For this review, use the dimensioned drawing (mm, ordinates from the lowest corner) and the shaded views. Coordinates: 2 decimals unless noted, no trailing zeros. Order: outer loops, then holes, each group sorted by start corner. A loop starts at its lowest first (then second) coordinate and runs counter-clockwise, first axis right, second up. Notation, with made-up numbers: M 80.25,69.25 L 103.25,69.25 A21 cw 103.25,86.25 Z; hole C 39.25,-10.75 d7. An arc over 180 degrees is marked long. One line per item, written item: value.
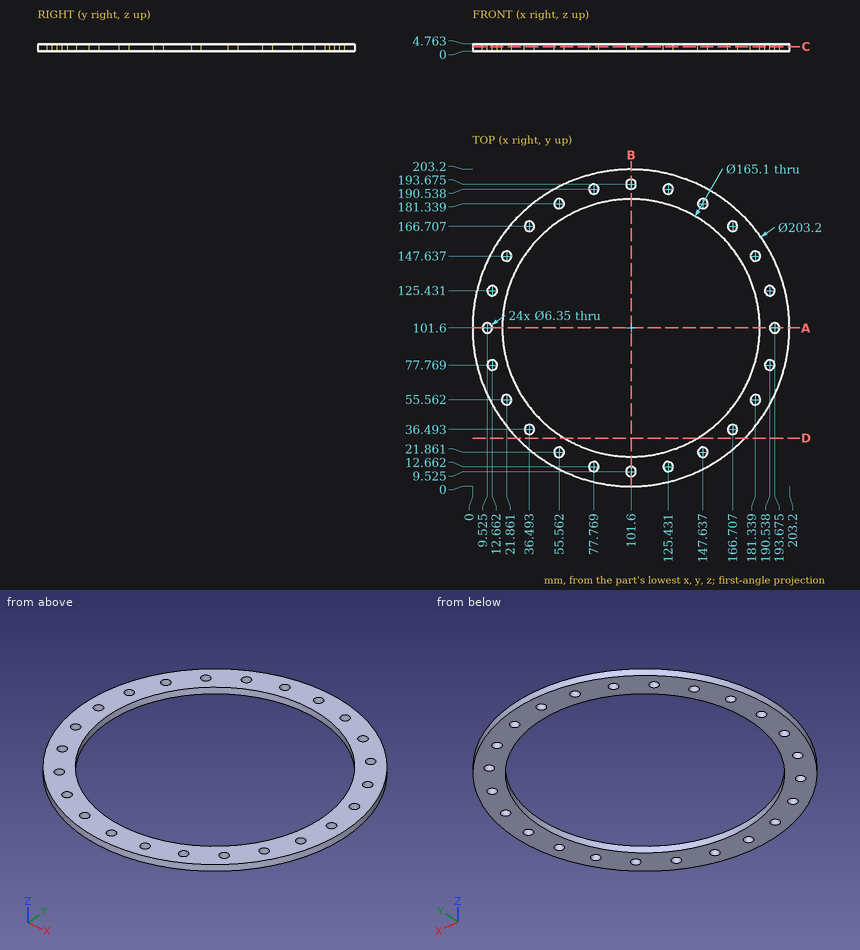
(1) We need section C-C, the plane z = 3.1. Count the separate pieces of the cut face and the enclosed holes in it, plus the area to 3 significant figures.
Geometry results:
separate pieces: 1
enclosed holes: 25
area: 10,300 mm2
(2) We need section A-A, the plane y = 101.6. State the section outline as (x, z) points, plus the area to 3 significant figures.
Geometry results:
outline: M 0,0 L 6.35,0 L 6.35,4.76 L 0,4.76 Z; M 12.7,0 L 19.05,0 L 19.05,4.76 L 12.7,4.76 Z; M 184.15,0 L 190.5,0 L 190.5,4.76 L 184.15,4.76 Z; M 196.85,0 L 203.2,0 L 203.2,4.76 L 196.85,4.76 Z
area: 121 mm2
(3) Insertion check: pin 1 Ø1.5 at (x, z) = (39, 1.5) entering from +Y (1 decimal). The pin has a flat end and moves straight along its axis. Give the tip position at first contact, or say it passes through.
Geometry results:
pin 1: stops at y = 182.2
(4) We need section D-D, the plane y = 31. State the section outline as (x, z) points.
Geometry results:
outline: M 28.54,0 L 58.82,0 L 58.82,4.76 L 28.54,4.76 Z; M 144.38,0 L 174.66,0 L 174.66,4.76 L 144.38,4.76 Z
(5) For L1, parallel to X at y = 145.5, z = 0.55 (1 decimal); L2, parallel to X at y = 102.5, z = 4.1 (1 decimal); L3, parallel to Y at x = 55, z = 3.5 (1 decimal), list the stretches that pass through material, from the lowest coordinate up.
Geometry results:
L1: x = 10 to 19.5, 24.2 to 31.7, 171.5 to 179, 183.7 to 193.2
L2: x = 0 to 6.5, 12.6 to 19.1, 184.1 to 190.6, 196.7 to 203.2
L3: y = 11.3 to 18.7, 25 to 33.5, 169.7 to 178.2, 184.5 to 191.9
